Here's how the part is built. I have some questions about the finished solid (model axes, mm). Coordinates: 2 decimals unless noted, no trailing zeros. Write each loop counter-clockwise with the first axis right and the second up, starting at its lowest first coordinate (ties: lowest second). Pieces come first, ordered by that corner, then holes. Notation, with made-up numbers: M 38,63.5 L 65,63.5 A21 cw 65,72.5 Z; hole C 55,56 d8. An arc over 180 degrees is marked long. Use a Markdown table: item, result.
```python
from build123d import *

# Parameters (mm, degrees)
F1_DEPTH = 3.175


with BuildPart() as f1:
    # F0 (on Right) → F1 (new body)
    with BuildSketch(Plane.YZ):
        Polygon((-155.575, 34.925), (-155.575, 12.7), (-158.75, 12.7), (-158.75, -12.7), (-155.575, -12.7), (-155.575, -34.925), (-142.039474, -34.925), (-142.039474, -38.1), (-125.328947, -38.1), (-125.328947, -34.925), (-108.618421, -34.925), (-108.618421, -38.1), (-95.25, -38.1), (-95.25, 12.7), (-19.05, 12.7), (-19.05, -34.925), (-8.355262, -34.925), (-8.355262, -38.1), (8.355264, -38.1), (8.355264, -34.925), (19.05, -34.925), (19.05, 12.7), (95.25, 12.7), (95.25, -38.1), (108.618422, -38.1), (108.618422, -34.925), (125.328949, -34.925), (125.328949, -38.1), (142.039475, -38.1), (142.039475, -34.925), (155.575, -34.925), (155.575, -12.7), (158.75, -12.7), (158.75, 12.7), (155.575, 12.7), (155.575, 34.925), (142.039475, 34.925), (142.039475, 38.1), (125.328949, 38.1), (125.328949, 34.925), (108.618422, 34.925), (108.618422, 38.1), (91.907896, 38.1), (91.907896, 34.925), (75.19737, 34.925), (75.19737, 38.1), (58.486843, 38.1), (58.486843, 34.925), (41.776317, 34.925), (41.776317, 38.1), (25.06579, 38.1), (25.06579, 34.925), (8.355264, 34.925), (8.355264, 38.1), (-8.355262, 38.1), (-8.355262, 34.925), (-25.065789, 34.925), (-25.065789, 38.1), (-41.776315, 38.1), (-41.776315, 34.925), (-58.486842, 34.925), (-58.486842, 38.1), (-75.197368, 38.1), (-75.197368, 34.925), (-91.907894, 34.925), (-91.907894, 38.1), (-108.618421, 38.1), (-108.618421, 34.925), (-125.328947, 34.925), (-125.328947, 38.1), (-142.039474, 38.1), (-142.039474, 34.925), align=None)
    extrude(amount=F1_DEPTH)


solid = f1.part
```
1. Suppose I cut it at A-A on z = -4.5. Write out the boundary of the cut face in (x, y) (3 decimals).
Answers follow:
| item | result |
|---|---|
| outline | M 0,-158.75 L 3.175,-158.75 L 3.175,-95.25 L 0,-95.25 Z; M 0,-19.05 L 3.175,-19.05 L 3.175,19.05 L 0,19.05 Z; M 0,95.25 L 3.175,95.25 L 3.175,158.75 L 0,158.75 Z |
2. Will these pins go through, and if not, where does the flat tip stop? pin 1 Ø1.6 at (x, y) = (1.5, -114.5) entering from +Z (3 decimals); pin 2 Ø1 at (x, y) = (1.5, 118.5) entering from -Z (3 decimals); pin 3 Ø1 at (x, z) = (1, 36) entering from -Y.
Answers follow:
| item | result |
|---|---|
| pin 1 | stops at z = 34.925 |
| pin 2 | stops at z = -34.925 |
| pin 3 | stops at y = -142.04 |
3. Suppose I cut it at C-C on z = 28.5. Write out the boundary of the cut face in (x, y) (3 decimals).
Answers follow:
| item | result |
|---|---|
| outline | M 0,-155.575 L 3.175,-155.575 L 3.175,155.575 L 0,155.575 Z |
4. I need wall thicknesses on probe 1 along Y at (x, z) = (2.5, -1.5); probe 2 along Y at (x, z) = (1.2, -33) (3 decimals); probe 3 along Y at (x, z) = (1.4, 25.5) (3 decimals). Which ranges of each line are inside material? Lowest first, please.
Answers follow:
| item | result |
|---|---|
| probe 1 | y = -158.75 to -95.25, -19.05 to 19.05, 95.25 to 158.75 |
| probe 2 | y = -155.575 to -95.25, -19.05 to 19.05, 95.25 to 155.575 |
| probe 3 | y = -155.575 to 155.575 |
5. Suppose I cut it at B-B on y = -52. Write out the boundary of the cut face in (x, z) (3 decimals), and give its area (3 significant figures).
Answers follow:
| item | result |
|---|---|
| outline | M 0,12.7 L 3.175,12.7 L 3.175,34.925 L 0,34.925 Z |
| area | 70.6 mm2 |
